Autodesk Inventor part; units mm, degrees
ref_plane "YZ Plane" through (0, 0, 0) normal (1, 0, 0) x (0, 1, 0)
ref_plane "XZ Plane" through (0, 0, 0) normal (0, 1, 0) x (-1, 0, 0)
ref_plane "XY Plane" through (0, 0, 0) normal (0, 0, 1) x (1, 0, 0)
sketch "Sketch1" plane through (0, 0, 0) normal (0, 0, 1) x (1, 0, 0)
  line L0 (0, 0) -> (0, -25) construction
  line L1 (6.25, 3) -> (6.25, -25)
  line L2 (6.25, -25) -> (10, -25)
  line L3 (10, -25) -> (10, 0)
  line L4 (0, 0) -> (6.25, 0) construction
  line L5 (10, 0) -> (21, 0)
  line L6 (21, 0) -> (21, 115)
  line L7 (8.25, 5) -> (16, 5)
  line L8 (16, 5) -> (16, 115)
  line L9 (21, 115) -> (16, 115)
  line L10 (0, 0) -> (0, 121) construction
  line L11 (6.25, 3) -> (8.25, 5)
  point P0 (6.25, 5)
  point P1 (3.125, 0)
  dimension "d0" = 12.5
  dimension "d1" = 20
  dimension "d2" = 25
  dimension "d6" = 115
  dimension "d8" = 5
  dimension "d9" = 5
  dimension "d11" = 32
  dimension "d16" = 2
  dimension "d17" = 2
revolve "Revolution1" add sketch "Sketch1" angle 360 about axis through (0, 0, 0) along (0, -1, 0)
thread "Thread1"
thread "Thread3"
properties part number "Lagertopf"
Read the model definition and answer for the solid it produces. Units are mm, in the model's axes. A direction names the side the tool comes from. Give positions to 0.01 mm unless a question says otherwise; leave off trailing zeros. Write each loop counter-clockwise with the first axis right and the second up, starting at its lowest first coordinate (ties: lowest second). Pieces come first, ordered by that corner, then holes. Notation, with made-up numbers: M 65,83 L 87,83 A22 cw 87,105 Z; hole C 82,0 d10. An arc over 180 degrees is marked long. Put each result on its own line as item: value. Start each with the question number.
1. For a pull along Z with two mould halves and no side action, classify faces 4 (the cylindrical face through (20.03, 58.3, -6.31)), 5 (the flat face through (4, -25, 5)), 6 (the conical face through (-5.059, 3.125, 3.879)) as released by +Z, released by -Z, zero draft, split by the parting line, or undercut.
2. The part is cut by section D-D, the plane z = 18. Give the vertices of the cut face in (x, y).
3. The part is cut by section C-C, the plane y = 56. Give the vertices of the cut face in (x, z), and give its area (3 significant figures).
4. The part is cut by section B-B, the plane z = 0. Give the vertices of the cut face in (x, y), and give its area (3 significant figures).
5. The part is cut by section A-A, the plane x = 0. Give the vertices of the cut face in (y, z), and give its area (3 significant figures).
6. Consider line 1 along Z through (x, y) = (0, -17); line 2 along Z through (x, y) = (0, 51); line 3 along Y through (x, z) = (-16, -6.5). Determine where each line is inside the solid, lowest interval first.
7. Which of the six approach directions +Z, -Z, +X, -X, +Y, -Y give full straight-line access (tool end or side, diameter ignored) to faces 1 (the cylindrical face through (-3.47, 60.77, 15.62)), 2 (the cylindrical face through (-2.17, -12.32, 9.76)), 3 (the cylindrical face through (5.96, -11.2, 1.88))?
8. Each of these flat-tipped pins is pushed along its axis until it touches: pin 1 Ø9.5 at (x, z) = (-4, 2) entering from +Y; pin 2 Ø5 at (x, y) = (8, 26.5) entering from -Z; pin 3 Ø1.5 at (x, y) = (-13, 42) entering from -Z. Where does it stop, or does it pass through?
Final values:
1. face 4: split by the parting line
1. face 5: zero draft
1. face 6: undercut
2. outline: M -10.82,0 L 10.82,0 L 10.82,115 L -10.82,115 Z
3. outline: C 0,0 d42; hole C 0,0 d32
3. area: 581 mm²
4. outline: M -21,0 L -10,0 L -10,-25 L -6.25,-25 L -6.25,3 L -8.25,5 L -16,5 L -16,115 L -21,115 Z; M 6.25,-25 L 10,-25 L 10,0 L 21,0 L 21,115 L 16,115 L 16,5 L 8.25,5 L 6.25,3 Z
4. area: 1,430 mm²
5. outline: M -25,-10 L 0,-10 L 0,-21 L 115,-21 L 115,-16 L 5,-16 L 5,-8.25 L 3,-6.25 L -25,-6.25 Z; M -25,6.25 L 3,6.25 L 5,8.25 L 5,16 L 115,16 L 115,21 L 0,21 L 0,10 L -25,10 Z
5. area: 1,430 mm²
6. line 1: z = -10 to -6.25, 6.25 to 10
6. line 2: z = -21 to -16, 16 to 21
6. line 3: y = 0 to 115
7. face 1: +Y
7. face 2: -Y
7. face 3: +Y, -Y
8. pin 1: stops at y = 5
8. pin 2: stops at z = -20.27
8. pin 3: stops at z = -17.06
